Here's how the part is built. I have some questions about the finished solid (model axes, mm). A direction names the side the tool comes from. Coordinates: 2 decimals unless noted, no trailing zeros. Order: outer loops, then holes, each group sorted by start corner. A loop starts at its lowest first (then second) coordinate and runs counter-clockwise, first axis right, second up. Notation, with made-up numbers: M 59,-32 L 76,-32 A20 cw 76,-13 Z; hole C -31,7 d2. An arc over 180 degrees is marked long. Answer as CSV lines item,"result". Start each with the question number.
```python
from build123d import *

# Parameters (mm, degrees)
BOSS_EXTRUDE1_DEPTH = 101.6
SKETCH2_R           = 5
CUT_EXTRUDE1_DEPTH  = 114.058535724


with BuildPart() as part:
    # Sketch1 → Boss-Extrude1 (new body)
    with BuildSketch(Plane(origin=(0, 0, 0), x_dir=(1, 0, 0), z_dir=(0, 1, 0))):
        Polygon((-12.7, 0), (12.7, 0), (12.7, -25.4), (16.7, -25.4), (16.7, 0), (38.1, 0), (38.1, 6.35), (-38.1, 6.35), (-38.1, 0), (-16.7, 0), (-16.7, -25.4), (-12.7, -25.4), align=None)
    extrude(amount=BOSS_EXTRUDE1_DEPTH)

    # Sketch2 → Cut-Extrude1 (cut, through all)
    with BuildSketch(Plane(origin=(0, 0, -6.35), x_dir=(-1, 0, 0), z_dir=(0, 0, -1))):
        with Locations((-25.4, 88.9)):
            Circle(SKETCH2_R)
        with Locations((25.4, 88.9)):
            Circle(SKETCH2_R)
        with Locations((-25.4, 12.7)):
            Circle(SKETCH2_R)
        with Locations((25.4, 12.7)):
            Circle(SKETCH2_R)
    extrude(amount=-CUT_EXTRUDE1_DEPTH, mode=Mode.SUBTRACT)


solid = part.part
```
1) Which directions (+Z, -Z, +X, -X, +Y, -Y) give clear straight access to the entire face, cutting with the end or side of a thin tool? Please do faces 1 (the face through (27, 50, 0)), 2 (the face through (1, 50, -6.35)), 3 (the face through (0, 0, -2)), 4 (the face through (-28, 50, 0)), 5 (the face through (12.7, 50, 13)).
2) Suppose I cut it at D-D on y = 61. Please give me the cut outline in (x, z), plus the area to 3 significant figures.
3) Suppose I cut it at C-C on z = 21. Please give me the cut outline in (x, y).
4) If we mould it in two halves opening along Y, with no side actions, what happens to faces 6 (the face through (-15, 50, 25.4)), 7 (the face through (26.051, 17.657, -3.219)), 8 (the face through (0, 101.6, -2)), 9 (the face through (-24.749, 17.657, -3.219))? For each: released by +Y, released by -Y, zero draft, split by the parting line, or undercut.
5) Suppose I cut it at B-B on y = 88.9. Please give me the cut outline in (x, z).
6) Will these pins go through, and if not, where does the flat tip stop? pin 1 Ø5 at (y, z) = (26.5, 9) entering from -X; pin 2 Ø11.5 at (x, y) = (-25.4, 12.7) entering from +Z; pin 3 Ø6 at (y, z) = (45.5, 5.5) entering from +X.
7) I need wall thicknesses on line 1 (Y direction, x = 25, z = -3); line 2 (X direction, y = 62, z = 24.5); line 3 (X direction, y = 12, z = -4). Which ranges of each line are inside material? Lowest first, please. Write a range as [from, to].
8) Suppose I cut it at A-A on x = -25.4. Please give me the cut outline in (y, z).
Output:
1,face 1,"+Z, +X, +Y, -Y"
1,face 2,"-Z, +X, -X, +Y, -Y"
1,face 3,"+Z, -Z, +X, -X, -Y"
1,face 4,"+Z, -X, +Y, -Y"
1,face 5,"+Z, +Y, -Y"
2,outline,"M -38.1,-6.35 L 38.1,-6.35 L 38.1,0 L 16.7,0 L 16.7,25.4 L 12.7,25.4 L 12.7,0 L -12.7,0 L -12.7,25.4 L -16.7,25.4 L -16.7,0 L -38.1,0 Z"
2,area,"687 mm²"
3,outline,"M -16.7,0 L -12.7,0 L -12.7,101.6 L -16.7,101.6 Z; M 12.7,0 L 16.7,0 L 16.7,101.6 L 12.7,101.6 Z"
4,face 6,"zero draft"
4,face 7,"undercut"
4,face 8,"released by +Y"
4,face 9,"undercut"
5,outline,"M -38.1,-6.35 L -30.4,-6.35 L -30.4,0 L -38.1,0 Z; M -20.4,-6.35 L 20.4,-6.35 L 20.4,0 L 16.7,0 L 16.7,25.4 L 12.7,25.4 L 12.7,0 L -12.7,0 L -12.7,25.4 L -16.7,25.4 L -16.7,0 L -20.4,0 Z; M 30.4,-6.35 L 38.1,-6.35 L 38.1,0 L 30.4,0 Z"
6,pin 1,"x = -16.7"
6,pin 2,"z = 0"
6,pin 3,"x = 16.7"
7,line 1,"[0, 7.72], [17.68, 83.92], [93.88, 101.6]"
7,line 2,"[-16.7, -12.7], [12.7, 16.7]"
7,line 3,"[-38.1, -30.35], [-20.45, 20.45], [30.35, 38.1]"
8,outline,"M 0,-6.35 L 7.7,-6.35 L 7.7,0 L 0,0 Z; M 17.7,-6.35 L 83.9,-6.35 L 83.9,0 L 17.7,0 Z; M 93.9,-6.35 L 101.6,-6.35 L 101.6,0 L 93.9,0 Z"
